from build123d import *

# Parameters (mm, degrees)
BOSS_EXTRUDE1_DEPTH = 36.449
SKETCH3_W           = 16.764
SKETCH3_H           = 1.905
BOSS_EXTRUDE3_DEPTH = 11.557
BOSS_EXTRUDE4_DEPTH = 11.43
CUT_EXTRUDE1_REACH  = 38.449


with BuildPart() as part:
    # Sketch1 → Boss-Extrude1 (new body)
    with BuildSketch(Plane.XY):
        Polygon((-1.524, 1.692251565), (-1.524, 13.249251565), (0.254, 13.249251565), (0.254, -0.085748435), (-20.066, -0.085748435), (-20.066, 13.249251565), (-18.288, 13.249251565), (-18.288, 1.692251565), align=None)
    extrude(amount=-BOSS_EXTRUDE1_DEPTH)

    # Sketch3 → Boss-Extrude3 (add)
    with BuildSketch(Plane(origin=(0, 1.692251565, 0), x_dir=(1, 0, 0), z_dir=(0, 1, 0))):
        with Locations((-9.906, 35.4965)):
            Rectangle(SKETCH3_W, SKETCH3_H)
    extrude(amount=BOSS_EXTRUDE3_DEPTH)

    # Sketch4 → Boss-Extrude4 (add)
    with BuildSketch(Plane(origin=(0, 13.249251565, 0), x_dir=(1, 0, 0), z_dir=(0, 1, 0))):
        Polygon((-9.906, 34.544), (0.254, 34.544), (0.254, 36.449), (-20.066, 36.449), (-20.066, 34.544), align=None)
    extrude(amount=BOSS_EXTRUDE4_DEPTH)

    # Sketch5 → Cut-Extrude1 (cut, up to next)
    with BuildSketch(Plane(origin=(0, 0, -36.449), x_dir=(-1, 0, 0), z_dir=(0, 0, -1)), mode=Mode.PRIVATE) as cut_extrude1_sk1:
        Polygon((9.906, 24.679251565), (14.351, 24.679251565), (14.351, 20.234251565), (5.461, 20.234251565), (5.461, 24.679251565), align=None)
    cut_extrude1_tool1 = extrude(cut_extrude1_sk1.sketch, amount=-CUT_EXTRUDE1_REACH, mode=Mode.PRIVATE) & part.part
    add(cut_extrude1_tool1.solids().sort_by_distance((-9.906, 22.456752, -36.449))[0], mode=Mode.SUBTRACT)


solid = part.part
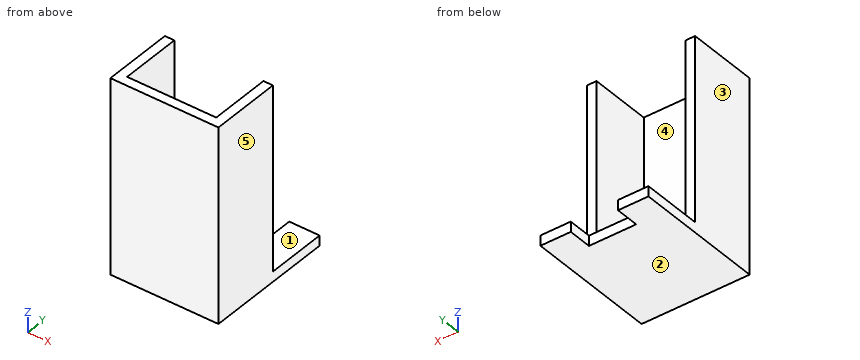
Input: part model. Units: mm. Frame: model coordinates. Face numbers are marked on the shaded views. A direction names the side the tool comes from. Round coordinates to 2 decimals unless told otherwise and drop trailing zeros. Order: outer loops, then holes, each group sorted by start corner. A loop starts at its lowest first (then second) coordinate and runs counter-clockwise, first axis right, second up.
1. Pin query (flat end, axial travel): P1, Ø6, axis at x = -13, y = 9, coming from the +Z side; P2, Ø2, axis at x = -0.5, z = -14.5, coming from the +Y side; P3, Ø4, axis at x = -7, z = -18.5, coming from the +Y side. Return the tip coordinate at first contact, or that it passes through.
The answers:
P1: stops at z = -34.54
P2: stops at y = 13.25
P3: stops at y = 1.69
2. Cut plane C-C, the plane x = -0.75. Output: boundary loops of the cut face in (y, z), then the cut area to 3 significant figures.
The answers:
outline: (-0.09, -36.45) - (24.68, -36.45) - (24.68, -34.54) - (13.25, -34.54) - (13.25, 0) - (-0.09, 0) - close
area: 508 mm2
3. Material intervals for line 1 (X direction, y = 8.75, z = -10.5); line 2 (Y direction, x = -14.75, z = -23); line 3 (Z direction, x = -14.75, y = 2.5), sorted ascending.
The answers:
line 1: x = -20.07 to -18.29, -1.52 to 0.25
line 2: y = -0.09 to 1.69
line 3: z = -36.45 to -34.54
4. Cut plane D-D, the plane x = -15.25. Output: boundary loops of the cut face in (y, z), then the cut area to 3 significant figures.
The answers:
outline: (-0.09, -36.45) - (24.68, -36.45) - (24.68, -34.54) - (1.69, -34.54) - (1.69, 0) - (-0.09, 0) - close
area: 109 mm2
5. Cut plane A-A, the plane z = -31. Output: boundary loops of the cut face in (x, y), then the cut area to 3 significant figures.
The answers:
outline: (-20.07, -0.09) - (0.25, -0.09) - (0.25, 13.25) - (-1.52, 13.25) - (-1.52, 1.69) - (-18.29, 1.69) - (-18.29, 13.25) - (-20.07, 13.25) - close
area: 77.2 mm2
6. Cut plane B-B, the plane y = 4.25. Output: boundary loops of the cut face in (x, z), then the cut area to 3 significant figures.
The answers:
outline: (-20.07, -36.45) - (0.25, -36.45) - (0.25, 0) - (-1.52, 0) - (-1.52, -34.54) - (-18.29, -34.54) - (-18.29, 0) - (-20.07, 0) - close
area: 162 mm2
7. Mould query, pull axis X, two halves, no side actions, for the marked faces 1, 2 and 3. Classes: released by +X, released by -X, zero draft, split by the parting line, or undercut.
The answers:
face 1: undercut
face 2: zero draft
face 3: released by -X
8. Set-up query: the marked faces 4 and 5. Return all of +Z, -Z, +X, -X, +Y, -Y with unobstructed straight access to the full face (end or side cutting, diameter ignored); none if empty.
The answers:
face 4: +Z, +Y
face 5: +Z, -Z, +X, +Y, -Y
